Part model, mm, in its own coordinate system. A direction names the side the tool comes from. Round coordinates to 2 decimals unless told otherwise and drop trailing zeros. Write each loop counter-clockwise with the first axis right and the second up, starting at its lowest first coordinate (ties: lowest second). Pieces come first, ordered by that corner, then holes. Notation, with made-up numbers: M 41.25,0.25 L 58.25,0.25 A13 cw 58.25,22.25 Z; hole C 51.25,13.5 d9. An arc over 180 degrees is marked long. Use a Markdown table: item, result. Add a question column.
1) Two-plate mould, pull along Y, no slides. Class faces 1 (the face through (-35, 0, 16)), 2 (the face through (-33, 18, 18)), 3 (the face through (-33.66, 22.11, 1.48)): released by +Y, released by -Y, zero draft, split by the parting line, or undercut.
2) Slice it at A-A on y = 12.5. Write the cut outline in (x, z), plus the area to 3 significant figures.
3) Slice it at C-C on x = -11. Give the number of separate pieces and of enclosed holes in the cut face, plus the area to 3 significant figures.
4) Which spindle directions (+Z, -Z, +X, -X, +Y, -Y) get a long thin tool onto all of the face, cutting with end or side? Do faces 4 (the face through (-45, 20, 1)), 5 (the face through (-32.581, 73.794, 0.493)), 6 (the face through (-45.535, 43.363, 17.493)). Say none if no direction does.
5) Wall check: probe 1 along Y at (x, z) = (-35, 1.75); probe 2 along Z at (x, y) = (-20, 75); probe 3 along X at (y, z) = (5, 2.15). Give the ranges that are in metal, low to high.
6) Drop flat-ended pins along their axis: P1, Ø1.5, axis at x = -6, z = 7, coming from the -Y side; P2, Ø0.8, axis at y = 29.5, z = 17.5, coming from the +X side; P3, Ø3, axis at x = -10, y = 70, coming from the +Z side; P4, Ø0.9, axis at x = -2, z = 6, coming from the -Y side. Give the stop position or say it passes through.
7) Slice it at B-B on z = 7.5. Write the cut outline in (x, y), plus the area to 4 significant figures.
```python
from build123d import *

# Parameters (mm, degrees)
ESQUISSE1_R                  = 2.5
BOSS_EXTRU_1_DEPTH           = 18
COQUE2_T                     = -3
ENL_V_MAT_EXTRU_1_DEPTH      = 94.536089292
ENL_V_MAT_EXTRU_1_DEPTH_BACK = 94.536089292
ESQUISSE2_W                  = 12
ESQUISSE2_H                  = 15
ESQUISSE3_R                  = 2.5
ENL_V_MAT_EXTRU_3_DEPTH      = 97.041657628
SHELL2_OUTLINE_R             = 4.5
SHELL2_DEPTH                 = 1
SHELL2_START                 = 17
SHELL2_2_OUTLINE_R           = 4.5
SHELL2_2_DEPTH               = 1


# Read off the part's stored shape, not the designer's step: Shell2
with BuildPart() as part:
    # Esquisse1 → Boss.-Extru.1 (new body)
    with BuildSketch(Plane.XY):
        Polygon((-50, 45), (-45, 40), (-45, 0), (-25, 0), (-25, 30), (0, 55), (0, 80), (-50, 80), align=None)
        with Locations((-35, 5)):
            Circle(ESQUISSE1_R, mode=Mode.SUBTRACT)
        with Locations((-35, 20)):
            Circle(ESQUISSE1_R, mode=Mode.SUBTRACT)
    extrude(amount=BOSS_EXTRU_1_DEPTH)

    # Coque2
    coque2_openings = [part.faces().sort_by_distance(p)[0] for p in [
        (-35, 0, 9),
        (-45, 20, 9),
        (-47.5, 42.5, 9),
        (-12.5, 42.5, 9),
        (-25, 15, 9),
        (-37.5, 5, 9),
        (-37.5, 20, 9),
    ]]
    offset(amount=COQUE2_T, openings=coque2_openings, kind=Kind.INTERSECTION)

    # Esquisse2 → Enlèv. mat.-Extru.1 (cut, two sides: drawn at the far end of the back side and taken through both)
    with BuildSketch(Plane.ZY.offset(45).offset(-ENL_V_MAT_EXTRU_1_DEPTH_BACK)):
        with Locations((9, 59.5)):
            Rectangle(ESQUISSE2_W, ESQUISSE2_H)
    extrude(amount=ENL_V_MAT_EXTRU_1_DEPTH + ENL_V_MAT_EXTRU_1_DEPTH_BACK, mode=Mode.SUBTRACT)

    # Esquisse3 → Enlèv. mat.-Extru.3 (cut, through all)
    with BuildSketch(Plane.XY.offset(18)):
        with Locations((-35, 70)):
            Circle(ESQUISSE3_R)
        with Locations((-10, 70)):
            Circle(ESQUISSE3_R)
    extrude(amount=-ENL_V_MAT_EXTRU_3_DEPTH, mode=Mode.SUBTRACT)

    # Shell2 outline → Shell2 (cut)
    with BuildSketch(Plane.XY):
        with BuildLine():
            Line((-43, 2), (-38.354101966, 2))
            ThreePointArc((-38.354101966, 2), (-35, 9.5), (-31.645898034, 2))
            Line((-31.645898034, 2), (-27, 2))
            Line((-27, 2), (-27, 30.828427125))
            Line((-27, 30.828427125), (-2, 55.828427125))
            Line((-2, 55.828427125), (-2, 78))
            Line((-2, 78), (-48, 78))
            Line((-48, 78), (-48, 45.828427125))
            Line((-48, 45.828427125), (-43, 40.828427125))
            Line((-43, 40.828427125), (-43, 2))
        make_face()
        with Locations((-35, 20)):
            Circle(SHELL2_OUTLINE_R, mode=Mode.SUBTRACT)
        with Locations((-35, 70)):
            Circle(SHELL2_OUTLINE_R, mode=Mode.SUBTRACT)
        with Locations((-10, 70)):
            Circle(SHELL2_OUTLINE_R, mode=Mode.SUBTRACT)
    extrude(amount=SHELL2_DEPTH, mode=Mode.SUBTRACT)

    # Shell2 2 outline → Shell2 2 (cut)
    with BuildSketch(Plane.XY.offset(SHELL2_START)):
        with BuildLine():
            Line((-43, 2), (-38.354101966, 2))
            ThreePointArc((-38.354101966, 2), (-35, 9.5), (-31.645898034, 2))
            Line((-31.645898034, 2), (-27, 2))
            Line((-27, 2), (-27, 30.828427125))
            Line((-27, 30.828427125), (-2, 55.828427125))
            Line((-2, 55.828427125), (-2, 78))
            Line((-2, 78), (-48, 78))
            Line((-48, 78), (-48, 45.828427125))
            Line((-48, 45.828427125), (-43, 40.828427125))
            Line((-43, 40.828427125), (-43, 2))
        make_face()
        with Locations((-35, 20)):
            Circle(SHELL2_2_OUTLINE_R, mode=Mode.SUBTRACT)
        with Locations((-35, 70)):
            Circle(SHELL2_2_OUTLINE_R, mode=Mode.SUBTRACT)
        with Locations((-10, 70)):
            Circle(SHELL2_2_OUTLINE_R, mode=Mode.SUBTRACT)
    extrude(amount=SHELL2_2_DEPTH, mode=Mode.SUBTRACT)


solid = part.part
```
Entries:
| question | item | result |
|---|---|---|
| 1 | face 1 | released by -Y |
| 1 | face 2 | zero draft |
| 1 | face 3 | undercut |
| 2 | outline | M -45,0 L -43,0 L -43,1 L -27,1 L -27,0 L -25,0 L -25,3 L -45,3 Z; M -45,15 L -25,15 L -25,18 L -27,18 L -27,17 L -43,17 L -43,18 L -45,18 Z |
| 2 | area | 88.0 mm^2 |
| 3 | separate pieces | 3 |
| 3 | enclosed holes | 0 |
| 3 | area | 180 mm^2 |
| 4 | face 4 | +Z, -Z, -X, -Y |
| 4 | face 5 | -Z |
| 4 | face 6 | +Z |
| 5 | probe 1 | y = 0 to 2.5, 7.5 to 17.5, 22.5 to 67.5, 72.5 to 80 |
| 5 | probe 2 | z = 1 to 3, 15 to 17 |
| 5 | probe 3 | x = -45 to -37.5, -32.5 to -25 |
| 6 | P1 | stops at y = 77 |
| 6 | P2 | stops at x = -25 |
| 6 | P3 | passes through |
| 6 | P4 | stops at y = 67 |
| 7 | outline | M -50,45 L -47,42 L -47,52 L -50,52 Z; M -50,67 L -47,67 L -47,77 L -3,77 L -3,67 L 0,67 L 0,80 L -50,80 Z |
| 7 | area | 235.5 mm^2 |
